Build history of the part. All positions in model axes, mm. A direction names the side the tool comes from. Give positions to 0.01 mm unless a question says otherwise; leave off trailing zeros. Loops run counter-clockwise (first coordinate to the right, second up) from the corner with the lowest first, then second, coordinate; pieces in that order, holes last. Notation, with made-up numbers: M 28.25,30.25 L 60.25,30.25 A13 ccw 60.25,47.25 Z; hole C -29,13.5 d1. An arc over 180 degrees is marked long. Answer as a JSON object with one key per item and string values. Group by question number.
1. Drill centre lines: line 1 along Y through (x, z) = (42, -14.5); line 2 along Z through (x, y) = (117, -28). Where is each one in solid material? Low to high. Write a range as [from, to].
2. Slice it at A-A (x = 16.5). List the corners of the cut face in (y, z).
3. Drop flat-ended pins along their axis: pin 1 Ø1.5 at (x, z) = (79, -12.5) entering from -Y; pin 2 Ø10 at (x, y) = (58, -25) entering from -Z. Give the stop position or say it passes through.
4. Slice it at B-B (y = -38.5). List the corners of the cut face in (x, z), then the cut area to 3 significant figures.
5. 3-axis set-ups, long thin cutter, end or side, ignore diameter. For faces 1 (the face through (45, -19, 1)), 2 (the face through (45, 23.027, -50)): which of +Z, -Z, +X, -X, +Y, -Y reach the whole face in a straight line?
6. Slice it at C-C (z = -51). List the corners of the cut face in (x, y), then the cut area to 3 significant figures.
from build123d import *

# Parameters (mm, degrees)
ESQUISSE1_W        = 58
ESQUISSE1_H        = 84.6
BOSS_EXTRU_1_DEPTH = 1
ESQUISSE2_W        = 58
ESQUISSE2_H        = 1
BOSS_EXTRU_2_DEPTH = 99
BOSS_EXTRU_3_DEPTH = 116


with BuildPart() as part:
    # Esquisse1 → Boss.-Extru.1 (new body)
    with BuildSketch(Plane.XY):
        with Locations((-11.490537589, -18.273098988)):
            Rectangle(ESQUISSE1_W, ESQUISSE1_H)
    extrude(amount=BOSS_EXTRU_1_DEPTH)

    # Esquisse2 → Boss.-Extru.2 (add)
    with BuildSketch(Plane(origin=(0, 0, 0), x_dir=(-1, 0, 0), z_dir=(0, 0, -1))):
        with Locations((11.490537589, 23.526901012)):
            Rectangle(ESQUISSE2_W, ESQUISSE2_H)
    extrude(amount=BOSS_EXTRU_2_DEPTH)

    # Esquisse3 → Boss.-Extru.3 (add)
    with BuildSketch(Plane(origin=(17.509462411, 0, 0), x_dir=(0, 0, -1), z_dir=(1, 0, 0))):
        Polygon((99, 24.026901012), (99, 23.026901012), (0, 23.026901012), (0, -60.573098988), (-1, -60.573098988), (-1, 24.026901012), align=None)
    extrude(amount=BOSS_EXTRU_3_DEPTH)


solid = part.part
Established:
{
 "1": {"line 1": "y = [23.03, 24.03]", "line 2": "z = [0, 1]"},
 "2": {"outline": "M -60.57,0 L 23.03,0 L 23.03,-99 L 24.03,-99 L 24.03,1 L -60.57,1 Z"},
 "3": {"pin 1": "stops at y = 23.03", "pin 2": "stops at z = 0"},
 "4": {"outline": "M -40.49,0 L 133.51,0 L 133.51,1 L -40.49,1 Z", "area": "174 mm^2"},
 "5": {"face 1": "+Z, +X, -X, +Y, -Y", "face 2": "-Z, +X, -X, -Y"},
 "6": {"outline": "M -40.49,23.03 L 133.51,23.03 L 133.51,24.03 L -40.49,24.03 Z", "area": "174 mm^2"}
}
